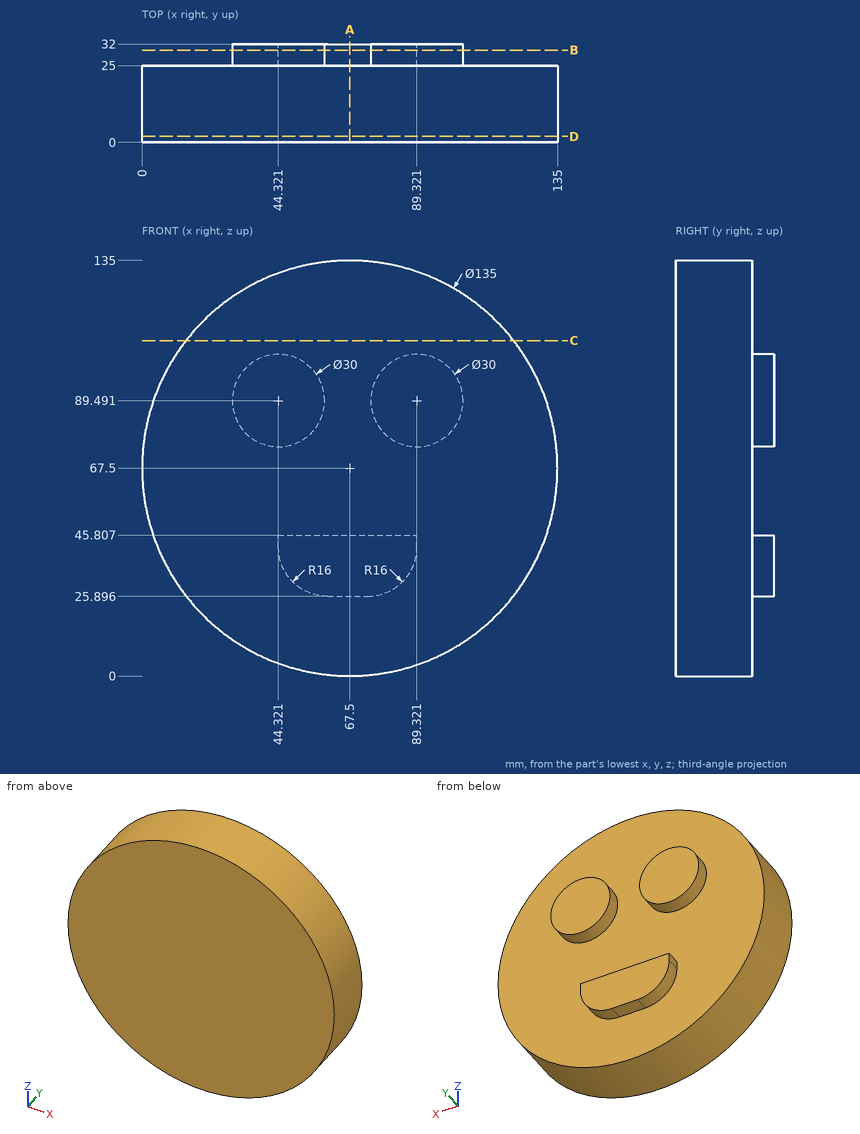
Drawing for the job (mm, zero at the part's lowest x, y, z). Coordinates: 2 decimals unless noted, no trailing zeros. Order: outer loops, then holes, each group sorted by start corner. A loop starts at its lowest first (then second) coordinate and runs counter-clockwise, first axis right, second up.
Item 1: Band-saw the part on B-B on y = 30. List the corners of the cut face in (x, z).
Check sheet entries:
outline: circle Ø30 at (44.32, 89.49); (44.32, 41.9) arc R16 ccw to (60.32, 25.9) - (73.32, 25.9) arc R16 ccw to (89.32, 41.9) - (89.32, 45.81) - (44.32, 45.81) - close; circle Ø30 at (89.32, 89.49)
Item 2: Band-saw the part on C-C on z = 109. List the corners of the cut face in (x, y) (1 decimal), plus the area to 3 significant figures.
Check sheet entries:
outline: (14.3, 0) - (120.7, 0) - (120.7, 25) - (14.3, 25) - close
area: 2,660 mm2
Item 3: Band-saw the part on D-D on y = 2. List the corners of the cut face in (x, z), plus the area to 3 significant figures.
Check sheet entries:
outline: circle Ø135 at (67.5, 67.5)
area: 14,300 mm2
Item 4: Drill centre lines: L1, parallel to Y at x = 47, z = 8; L2, parallel to X at y = 27, z = 92; L3, parallel to Z at x = 17, y = 8. Where is each one in solid material? Low to high.
Check sheet entries:
L1: y = 0 to 25
L2: x = 29.53 to 59.11, 74.53 to 104.11
L3: z = 22.71 to 112.29
Item 5: Band-saw the part on A-A on x = 67.5. List the corners of the cut face in (y, z), plus the area to 3 significant figures.
Check sheet entries:
outline: (0, 0) - (25, 0) - (25, 25.9) - (32, 25.9) - (32, 45.81) - (25, 45.81) - (25, 135) - (0, 135) - close
area: 3,510 mm2
Item 6: Pin check, flat tips, straight feed: pin 1 Ø10 at (x, y) = (27, 11.5) entering from -Z; pin 2 Ø2 at (x, y) = (76, 28) entering from +Z (1 decimal); pin 3 Ø1 at (x, z) = (67.5, 81) entering from +Y. Stop position of each tip, or through.
Check sheet entries:
pin 1: stops at z = 10.09
pin 2: stops at z = 98
pin 3: stops at y = 25
